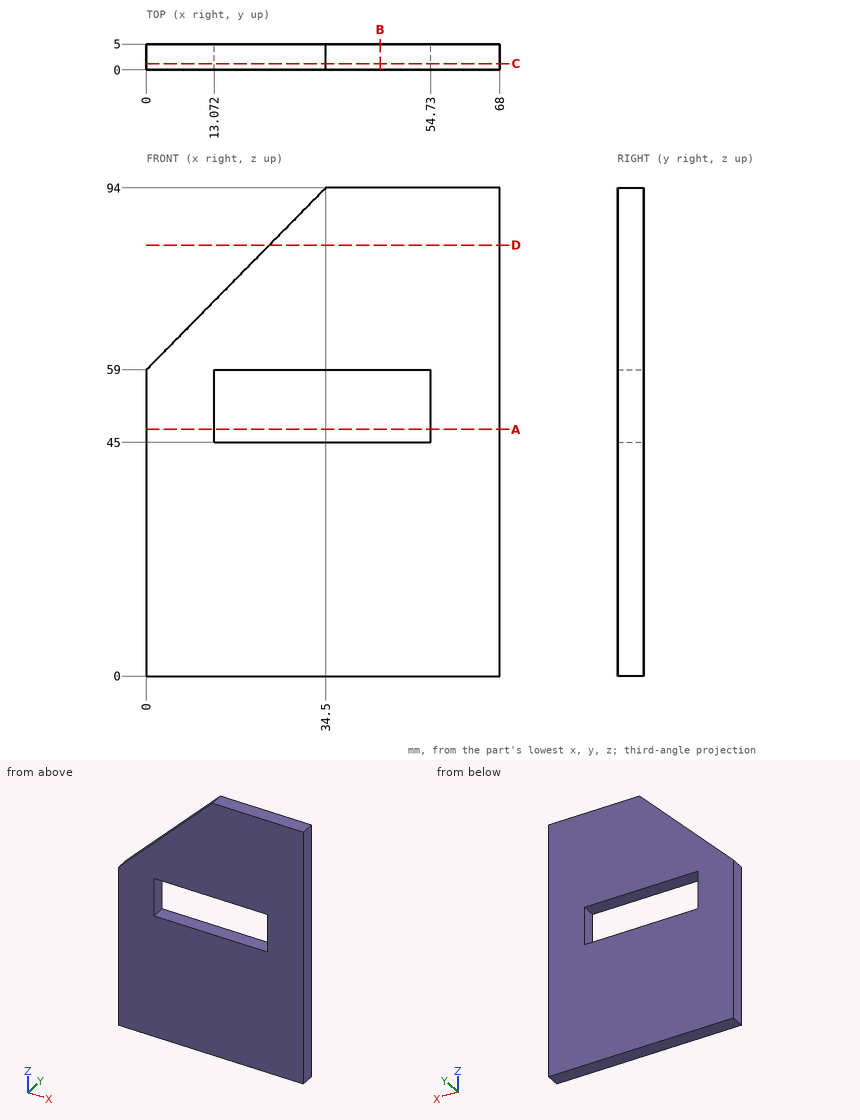
Drawing for the job (mm, zero at the part's lowest x, y, z). Round coordinates to 2 decimals unless told otherwise and drop trailing zeros. Loops run counter-clockwise (first coordinate to the right, second up) from the corner with the lowest first, then second, coordinate; pieces in that order, holes last. Notation, with made-up numbers: (21.5, 81.5) -> (27.5, 81.5) arc R18 ccw to (27.5, 102.5) -> close; hole circle Ø1 at (61.5, -13). An arc over 180 degrees is marked (long way). Use one line per item in the form item = value. Start each with the question number.
Item 1: Drill centre lines: line 1 along X through (y, z) = (3.4, 51); line 2 along Z through (x, y) = (46, 1.45); line 3 along Z through (x, y) = (19, 0.6) (1 decimal). Where is each one in solid material? Low to high.
Item 2: Band-saw the part on C-C (y = 1.2). List the corners of the cut face in (x, z).
Item 3: Band-saw the part on D-D (z = 83). List the corners of the cut face in (x, y), plus the area to 3 significant figures.
Item 4: Band-saw the part on B-B (x = 45). List the corners of the cut face in (y, z), plus the area to 3 significant figures.
Item 5: Band-saw the part on A-A (z = 47.5). List the corners of the cut face in (x, y).
Item 6: Drop flat-ended pins along their axis: pin 1 Ø5 at (x, z) = (17.5, 54) entering from +Y; pin 2 Ø1.5 at (x, y) = (34, 2.5) entering from -Z; pin 3 Ø2 at (y, z) = (1, 71.5) entering from -X (1 decimal); pin 4 Ø3 at (x, y) = (15, 4.5) entering from +Z. Give the stop position or say it passes through.
Data:
q1.line_1 = 0 to 13.07, 54.73 to 68
q1.line_2 = 0 to 45, 59 to 94
q1.line_3 = 0 to 45, 59 to 78.3
q2.outline = (0, 0) -> (68, 0) -> (68, 94) -> (34.5, 94) -> (0, 59) -> close; hole (13.07, 45) -> (54.73, 45) -> (54.73, 59) -> (13.07, 59) -> close
q3.outline = (23.66, 0) -> (68, 0) -> (68, 5) -> (23.66, 5) -> close
q3.area = 222 mm^2
q4.outline = (0, 0) -> (5, 0) -> (5, 45) -> (0, 45) -> close; (0, 59) -> (5, 59) -> (5, 94) -> (0, 94) -> close
q4.area = 400 mm^2
q5.outline = (0, 0) -> (13.07, 0) -> (13.07, 5) -> (0, 5) -> close; (54.73, 0) -> (68, 0) -> (68, 5) -> (54.73, 5) -> close
q6.pin_1 = through
q6.pin_2 = 0
q6.pin_3 = 11.3
q6.pin_4 = 75.74
